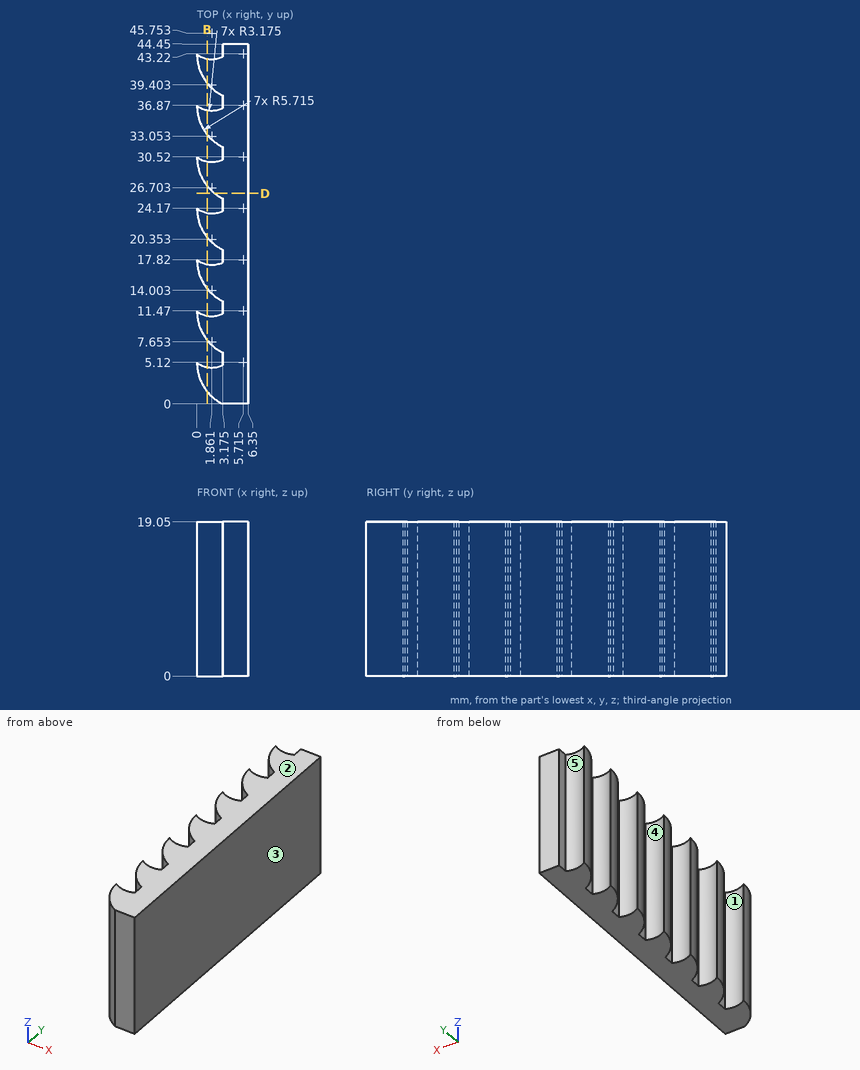
Geometry check sheet. Reference: drawing and pictorial views, mm from the part's lowest x, y, z. A direction names the side the tool comes from. Round coordinates to 2 decimals unless told otherwise and drop trailing zeros. Loops run counter-clockwise (first coordinate to the right, second up) from the corner with the lowest first, then second, coordinate; pieces in that order, holes last.
1. Sectioned sample at D-D on y = 26. Record the boundary of the cut face in (x, z).
2. Mould release check, pull along Y, two halves, no side actions. Record for the marked faces 3, 4 and 5: released by +Y, released by -Y, zero draft, split by the parting line, or undercut.
3. Scan lines: probe 1 along X at (y, z) = (9, 18); probe 2 along X at (y, z) = (10, 9.75). Record each from-to range of solid material in increasing order.
4. Gauge pin test, flat ends, axial feed: pin 1 Ø0.8 at (y, z) = (18.5, 10.5) entering from -X (3 decimals); pin 2 Ø1 at (y, z) = (10.5, 8.5) entering from -X; pin 3 Ø0.8 at (y, z) = (6, 7.5) entering from -X (1 decimal). Record the tip position at first contact, or that the pin passes through.
5. Set-up check for the marked faces 1 and 2: record each of +Z, -Z, +X, -X, +Y, -Y from which the full face is reachable in a straight line by a thin tool's end or side.
6. Sectioned sample at B-B on x = 1.25. Record the boundary of the cut face in (y, z).
Recorded:
1. outline: (2.22, 0) - (6.35, 0) - (6.35, 19.05) - (2.22, 19.05) - close
2. face 3: zero draft
2. face 4: undercut
2. face 5: released by +Y
3. probe 1: x = 0.56 to 6.35
3. probe 2: x = 0.19 to 6.35
4. pin 1: stops at x = 3.175
4. pin 2: stops at x = 0.02
4. pin 3: stops at x = 3.1
5. face 1: +Z, -Z
5. face 2: +Z, +X, -X, +Y, -Y
6. outline: (1.55, 0) - (4.54, 0) - (4.54, 19.05) - (1.55, 19.05) - close; (7.9, 0) - (10.89, 0) - (10.89, 19.05) - (7.9, 19.05) - close; (14.25, 0) - (17.24, 0) - (17.24, 19.05) - (14.25, 19.05) - close; (20.6, 0) - (23.59, 0) - (23.59, 19.05) - (20.6, 19.05) - close; (26.95, 0) - (29.94, 0) - (29.94, 19.05) - (26.95, 19.05) - close; (33.3, 0) - (36.29, 0) - (36.29, 19.05) - (33.3, 19.05) - close; (39.65, 0) - (42.64, 0) - (42.64, 19.05) - (39.65, 19.05) - close
